from build123d import *

# Parameters (mm, degrees)
SALIENTE_EXTRUIR1_DEPTH = 15
CROQUIS2_R              = 3.2
CORTAR_EXTRUIR1_DEPTH   = 10.75
CORTAR_EXTRUIR2_START   = -3
CORTAR_EXTRUIR2_DEPTH   = 7.75
CHAFL_N1_SIZE           = 2


with BuildPart() as part:
    # Croquis1 → Saliente-Extruir1 (new body, symmetric)
    with BuildSketch(Plane(origin=(0, 0, 0), x_dir=(1, 0, 0), z_dir=(0, 1, 0))):
        Polygon((0, 0), (-30, 0), (-30, 8), (-1.75, 8), (0, 9.75), (9.4, 9.75), (9.4, 1.75), (0, 1.75), align=None)
    extrude(amount=SALIENTE_EXTRUIR1_DEPTH, both=True)

    # Croquis2 → Cortar-Extruir1 (cut, through all)
    with BuildSketch(Plane.XY):
        with Locations((-15, 0)):
            Circle(CROQUIS2_R)
    extrude(amount=-CORTAR_EXTRUIR1_DEPTH, mode=Mode.SUBTRACT)

    # Croquis3 → Cortar-Extruir2 (cut, through all)
    with BuildSketch(Plane.XY.offset(CORTAR_EXTRUIR2_START)):
        Polygon((-9.226497308, 0), (-12.113248654, 5), (-17.886751346, 5), (-20.773502692, 0), (-17.886751346, -5), (-12.113248654, -5), align=None)
    extrude(amount=-CORTAR_EXTRUIR2_DEPTH, mode=Mode.SUBTRACT)

    # Chaflán1
    chafl_n1_edges = [part.edges().sort_by_distance(p)[0] for p in [
        (9.4, 0, -9.75),
        (9.4, 0, -1.75),
        (-30, 15, -4),
        (-30, -15, -4),
    ]]
    chamfer(chafl_n1_edges, length=CHAFL_N1_SIZE)


solid = part.part
Geometry: final body of the model. Coordinates: model frame, mm. A direction names the side the tool comes from. Coordinates: 2 decimals unless noted, no trailing zeros. Order: outer loops, then holes, each group sorted by start corner. A loop starts at its lowest first (then second) coordinate and runs counter-clockwise, first axis right, second up.
1) Section B-B (z = -6.25). Return loops of the section in (x, y), then the cut area to 3 significant figures.
Result sheet:
outline: (-30, -13) - (-28, -15) - (9.4, -15) - (9.4, 15) - (-28, 15) - (-30, 13) - close; hole (-20.77, 0) - (-17.89, -5) - (-12.11, -5) - (-9.23, 0) - (-12.11, 5) - (-17.89, 5) - close
area: 1,090 mm2
2) Section D-D (z = -2.5). Return loops of the section in (x, y).
Result sheet:
outline: (-30, -13) - (-28, -15) - (8.15, -15) - (8.15, 15) - (-28, 15) - (-30, 13) - close; hole circle Ø6.4 at (-15, 0)
3) Draft query along X for faces 4 (the flat face through (9.4, 0, -6)), 5 (the flat face through (-15, -5, -5)), 6 (the flat face through (4, 0, -9.75)). Return one class per face: released by +X, released by -X, zero draft, split by the parting line, or undercut.
Result sheet:
face 4: released by +X
face 5: undercut
face 6: zero draft
4) First-contact query: P1, Ø8, axis at x = 5, y = -1.5, coming from the +Z side; P2, Ø6, axis at x = -15, y = 0, coming from the +Z side; P3, Ø0.5, axis at y = 3.5, z = -1, coming from the +X side; P4, Ø14, axis at x = -10, y = 7, coming from the -Z side. Flat tips, straight axial feed; report the tip coordinate or a pass-through.
Result sheet:
P1: stops at z = -1.75
P2: passes through
P3: stops at x = 0
P4: stops at z = -8
5) Ray query, probe 1 along Y at (x, z) = (-15, -1.05); probe 2 along Z at (x, y) = (-8, -6.75); probe 3 along X at (y, z) = (1.75, -3.25). Return the intervals inside material, ascending.
Result sheet:
probe 1: y = -15 to -3.2, 3.2 to 15
probe 2: z = -8 to 0
probe 3: x = -30 to -19.76, -10.24 to 8.9
6) Set-up query: faces 1 (the flat face through (-10.65, 2.465, -5.465)), 2 (the flat face through (4, 0, -1.75)), 3 (the flat face through (-0.89, 0.21, -8.86)). Return all of +Z, -Z, +X, -X, +Y, -Y with unobstructed straight access to the full face (end or side cutting, diameter ignored); none if empty.
Result sheet:
face 1: -Z
face 2: +Z, +X, +Y, -Y
face 3: -Z, -X, +Y, -Y
7) Section A-A (x = -15). Return loops of the section in (y, z), then the cut area to 3 significant figures.
Result sheet:
outline: (-15, -8) - (-5, -8) - (-5, -3) - (-3.2, -3) - (-3.2, 0) - (-15, 0) - close; (3.2, -3) - (5, -3) - (5, -8) - (15, -8) - (15, 0) - (3.2, 0) - close
area: 171 mm2
8) Section C-C (y = 6.25). Return loops of the section in (x, z).
Result sheet:
outline: (-30, -8) - (-1.75, -8) - (0, -9.75) - (7.4, -9.75) - (9.4, -7.75) - (9.4, -3.75) - (7.4, -1.75) - (0, -1.75) - (0, 0) - (-30, 0) - close
